from build123d import *

# Parameters (mm, degrees)
BOSS_EXTRUDE1_DEPTH = 3
SKETCH2_W           = 191
SKETCH2_H           = 40
CUT_EXTRUDE1_DEPTH  = 4
FILLET1_R           = 3
SKETCH3_W           = 3
SKETCH3_H           = 10
CUT_EXTRUDE2_DEPTH  = 4
FILLET2_R           = 4
BOSS_EXTRUDE2_DEPTH = 3


with BuildPart() as part:
    # Sketch1 → Boss-Extrude1 (new body)
    with BuildSketch(Plane.XY):
        Polygon((-16, 19.999811529), (16, 19.999811529), (113.979628183, 0), (113.979628183, -25), (-113.979628183, -25), (-113.979628183, 0), align=None)
    extrude(amount=BOSS_EXTRUDE1_DEPTH)

    # Sketch2 → Cut-Extrude1 (cut, through all)
    with BuildSketch(Plane.XY.offset(3)):
        with Locations((0, -25)):
            Rectangle(SKETCH2_W, SKETCH2_H)
    extrude(amount=-CUT_EXTRUDE1_DEPTH, mode=Mode.SUBTRACT)

    # Fillet1
    fillet1_edges = [part.edges().sort_by_distance(p)[0] for p in [
        (95.5, -5, 1.5),
        (-95.5, -5, 1.5),
    ]]
    fillet(fillet1_edges, radius=FILLET1_R)

    # Sketch3 → Cut-Extrude2 (cut, through all)
    with BuildSketch(Plane.XY.offset(3)):
        with Locations((-61.5, -5)):
            Rectangle(SKETCH3_W, SKETCH3_H)
        with Locations((61.5, -5)):
            Rectangle(SKETCH3_W, SKETCH3_H)
    extrude(amount=-CUT_EXTRUDE2_DEPTH, mode=Mode.SUBTRACT)

    # Fillet2
    fillet2_edges = [part.edges().sort_by_distance(p)[0] for p in [
        (113.979628183, -25, 1.5),
        (-113.979628183, -25, 1.5),
    ]]
    fillet(fillet2_edges, radius=FILLET2_R)

    # Sketch4 → Boss-Extrude2 (add)
    with BuildSketch(Plane.XY.offset(3)):
        Polygon((-26.29440044, 17.898496465), (0, 23.265765793), (26.811324143, 17.792980892), align=None)
    extrude(amount=-BOSS_EXTRUDE2_DEPTH)


solid = part.part
Part model, mm, in its own coordinate system. Give positions to 0.01 mm unless a question says otherwise; leave off trailing zeros. Loops run counter-clockwise (first coordinate to the right, second up) from the corner with the lowest first, then second, coordinate; pieces in that order, holes last.
(1) Drill centre lines: line 1 along X through (y, z) = (-3, 0.3); line 2 along X through (y, z) = (-16, 1.8); line 3 along Y through (x, z) = (40, 2.65). Where is each one in solid material? Low to high.
Return value:
line 1: x = -113.98 to -63, -60 to 60, 63 to 113.98
line 2: x = -113.98 to -95.5, 95.5 to 113.98
line 3: y = -5 to 15.1
(2) Band-saw the part on A-A (y = -2). Write the cut outline in (x, z), and give its area (3 significant figures).
Return value:
outline: (-113.98, 0) - (-63, 0) - (-63, 3) - (-113.98, 3) - close; (-60, 0) - (60, 0) - (60, 3) - (-60, 3) - close; (63, 0) - (113.98, 0) - (113.98, 3) - (63, 3) - close
area: 666 mm2
(3) Band-saw the part on D-D (y = 10). Write the cut outline in (x, z), and give its area (3 significant figures).
Return value:
outline: (-64.99, 0) - (64.99, 0) - (64.99, 3) - (-64.99, 3) - close
area: 390 mm2
(4) Band-saw the part on C-C (x = 25). Write the cut outline in (y, z).
Return value:
outline: (-5, 0) - (18.16, 0) - (18.16, 3) - (-5, 3) - close
(5) Band-saw the part on B-B (z = 0.5). Write the cut outline in (x, y), and give its area (3 significant figures).
Return value:
outline: (-113.98, -21) arc R4 ccw to (-109.98, -25) - (-95.5, -25) - (-95.5, -8) arc R3 cw to (-92.5, -5) - (-63, -5) - (-63, 0) - (-60, 0) - (-60, -5) - (60, -5) - (60, 0) - (63, 0) - (63, -5) - (92.5, -5) arc R3 cw to (95.5, -8) - (95.5, -25) - (109.98, -25) arc R4 ccw to (113.98, -21) - (113.98, 0) - (0, 23.27) - (-113.98, 0) - close
area: 4,500 mm2
(6) Pin check, flat tips, straight feed: pin 1 (1.5 mm diameter, centred on x = 80, z = 1, fed in from -Y); pin 2 (0.9 mm diameter, centred on x = -61, z = 1, fed in from -Y). Stop position of each tip, or through.
Return value:
pin 1: stops at y = -5
pin 2: stops at y = 0
